from build123d import *

# Parameters (mm, degrees)
F0_R          = 25
F0_R_2        = 23
F1_DEPTH      = 310
F7_R          = 25
F7_R_2        = 23
F8_DEPTH      = 200
F8_DEPTH_BACK = 25


with BuildPart() as f1:
    # F0 (on Front) → F1 (new body)
    with BuildSketch(Plane.XZ):
        Circle(F0_R)
        Circle(F0_R_2, mode=Mode.SUBTRACT)
    extrude(amount=F1_DEPTH)

    # F7 (on line) → F8 (join, two sides)
    with BuildSketch(Plane(origin=(69.9519052838, -121.1602540378, 0), x_dir=(-0.8660254038, -0.5, 0), z_dir=(-0.5, 0.8660254038, 0))) as f8_sk:
        with Locations((57.6794919243, 0)):
            Circle(F7_R)
        with Locations((57.6794919243, 0)):
            Circle(F7_R_2, mode=Mode.SUBTRACT)
    extrude(amount=-F8_DEPTH)
    extrude(f8_sk.sketch, amount=F8_DEPTH_BACK)


solid = f1.part
Can you work these out from the model? Positions are in its coordinate system, mm. A direction names the side the tool comes from. Round coordinates to 2 decimals unless told otherwise and drop trailing zeros. Loops run counter-clockwise (first coordinate to the right, second up) from the corner with the lowest first, then second, coordinate; pieces in that order, holes last. Notation, with made-up numbers: (2.25, 6) - (22.25, 6) arc R12 ccw to (22.25, 29) - close; hole circle Ø10 at (36.25, 34). An arc over 180 degrees is marked (long way). Write item = value, one per line. Start each with the question number.
(1) If we section it at B-B (y = -106): Please give me the cut outline in (x, z).
(2) For P1, Ø10, axis at x = 98, y = -255, coming from the -Z side; P2, Ø8, axis at x = 22.5, y = -239, coming from the +Z side; P3, Ø12, axis at x = 84, z = 0, coming from the +Y side, each with a flat end and sliding along its axis, tell me the tip position at first contact or that it passes through.
(3) If we section it at C-C (z = 0): Please give me the cut outline in (x, y).
(4) If we mould it in two halves opening along X, with no side actions, what happens to faces 4 (the face through (22.1, 0, -7.3)), 5 (the face through (100.856, -334.258, -7.291)), 6 (the face through (86.167, -214.653, 1.099))? For each: released by +X, released by -X, zero draft, split by the parting line, or undercut.
(5) For faces 1 (the face through (22.1, -310, -7.3)), 2 (the face through (-2.994, -152.83, 22.804)), 3 (the face through (-13.099, -140.242, 0.107)), which set-ups out of +Z, -Z, +X, -X, +Y, -Y let a thin tool reach every point of the face, with its end or its side?
(6) If I drill on probe 1 along Z at (x, y) = (0, -231); probe 2 along X at (y, z) = (-274, 5.5); probe 3 along X at (y, z) = (-250, -13), over which ranges is the centre line in solid material (lowest first)? Write a range as [from, to].
(7) If we section it at A-A (z = 13.5): Please give me the cut outline in (x, y).
Ans:
q1.outline = circle Ø50 at (0, 0); hole circle Ø46 at (0, 0)
q2.P1 = -22.89
q2.P2 = 16.82
q2.P3 = -200.46
q3.outline = (-25, -310) - (-23, -310) - (-23, 0) - (-25, 0) - close; (-14.15, -140.85) - (23, -205.2) - (23, -310) - (25, -310) - (25, -208.66) - (98.35, -335.71) - (100.08, -334.71) - (25, -204.66) - (25, 0) - (23, 0) - (23, -201.2) - (-12.42, -139.85) - close; (27.42, -116.85) - (139.92, -311.71) - (141.65, -310.71) - (29.15, -115.85) - close
q4.face_4 = zero draft
q4.face_5 = released by +X
q4.face_6 = undercut
q5.face_1 = +Z, -Z, -X, -Y
q5.face_2 = none
q5.face_3 = +Y
q6.probe_1 = [-25, -23], [23, 25]
q6.probe_2 = [-24.39, -22.33], [22.33, 24.39], [63.43, 65.8], [117.38, 119.75]
q6.probe_3 = [-21.35, -18.97], [18.97, 21.35], [53.08, 55.83], [99.64, 102.39]
q7.outline = (-21.04, -310) - (-18.62, -310) - (-18.62, 0) - (-21.04, 0) - close; (-10.72, -138.87) - (18.62, -189.7) - (18.62, -310) - (21.04, -310) - (21.04, -193.89) - (101.78, -333.73) - (103.87, -332.52) - (21.04, -189.05) - (21.04, 0) - (18.62, 0) - (18.62, -184.85) - (-8.63, -137.66) - close; (23.63, -119.04) - (136.13, -313.89) - (138.22, -312.68) - (25.72, -117.83) - close
